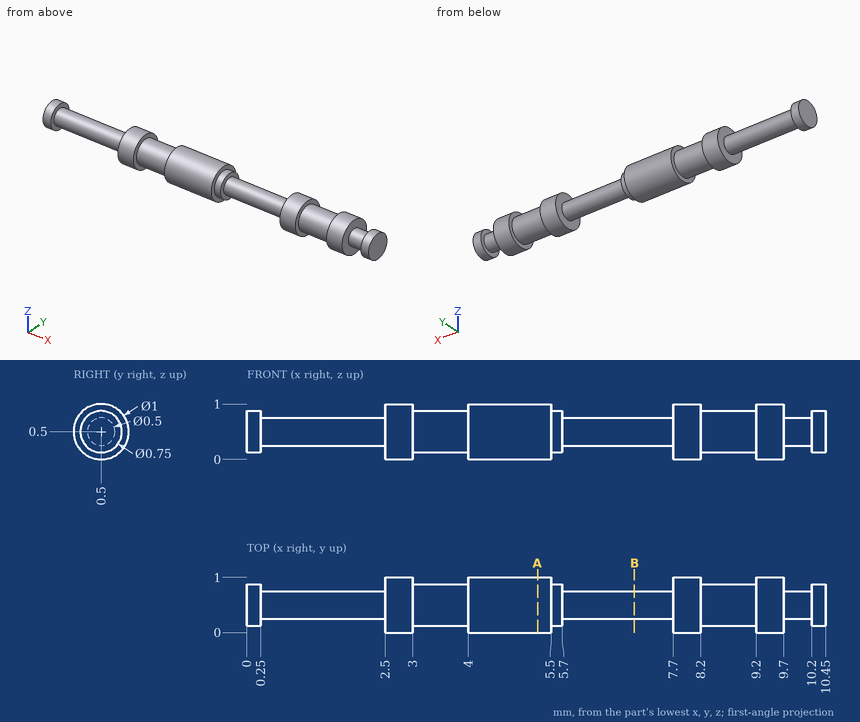
Drawing for the job (mm, zero at the part's lowest x, y, z). Round coordinates to 2 decimals unless told otherwise and drop trailing zeros. Write each loop counter-clockwise with the first axis right and the second up, starting at its lowest first coordinate (ties: lowest second). Pieces come first, ordered by that corner, then holes. Notation, with made-up numbers: M 85,88.5 L 136,88.5 A33 cw 136,126.5 Z; hole C -16.5,61.25 d4. An arc over 180 degrees is marked long. Answer as a JSON object with one key per item and string values. Group by question number.
(1) Cut at A-A (x = 5.25). Give the cut face in (y, z), and give its area (3 significant figures).
(2) Drill centre lines: L1, parallel to X at y = 0.85, z = 0.75; L2, parallel to X at y = 0.55, z = 0.2; L3, parallel to Z at x = 9.25, y = 0.45. Where is each one in solid material? Low to high.
(3) Cut at B-B (x = 7). Give the cut face in (y, z).
Responses:
{
 "1": {"outline": "C 0.5,0.5 d1", "area": "0.785 mm2"},
 "2": {"L1": "x = 2.5 to 3, 4 to 5.5, 7.7 to 8.2, 9.2 to 9.7", "L2": "x = 0 to 0.25, 2.5 to 5.7, 7.7 to 9.7, 10.2 to 10.45", "L3": "z = 0 to 1"},
 "3": {"outline": "C 0.5,0.5 d0.5"}
}
